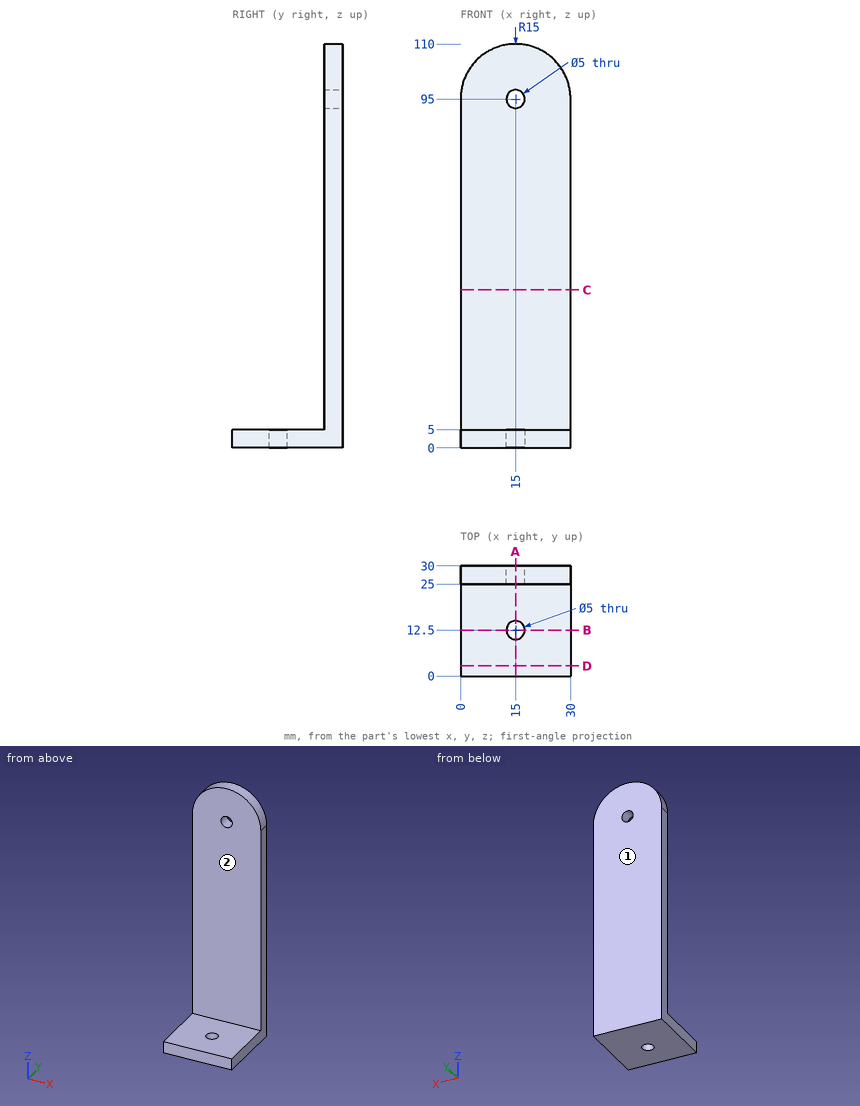
Can you work these out from the drawing? Everything is in mm from the part's minimum corner. A direction names the side the tool comes from. Give positions to 0.01 mm unless a question says otherwise; leave off trailing zeros. Loops run counter-clockwise (first coordinate to the right, second up) from the corner with the lowest first, then second, coordinate; pieces in that order, holes last. Notation, with made-up numbers: M 36,71.25 L 92,71.25 A32 cw 92,100.25 Z; hole C 44.25,77.25 d5. An arc over 180 degrees is marked long. Use CSV: the item, a comma, the result in double quotes. Start each with the question number.
1. On a 3-axis mill with a long thin cutter (end or side, diameter ignored), from which of +Z, -Z, +X, -X, +Y, -Y can I reach the whole of each face in a straight line? I mean the marked faces 1 and 2. Say none if no direction works.
2. For P1, Ø4, axis at x = 14.5, y = 19, coming from the +Z side; P2, Ø6.5, axis at x = 15, z = 95, coming from the -Y side; P3, Ø6, axis at x = 26.5, y = 3, coming from the -Z side, each with a flat end and sliding along its axis, tell me the tip position at first contact or that it passes through.
3. Imagine slicing it at C-C, the plane z = 43. Write out the boundary of the cut face in (x, y).
4. Imagine slicing it at B-B, the plane y = 12.5. Write out the boundary of the cut face in (x, z).
5. Imagine slicing it at D-D, the plane y = 2.75. Write out the boundary of the cut face in (x, z), plus the area to 3 significant figures.
6. Imagine slicing it at A-A, the plane x = 15. Write out the boundary of the cut face in (y, z).
7. If I drill on L1, parallel to Z at x = 15, y = 27.75; L2, parallel to Y at x = 15, z = 2.5; L3, parallel to X at y = 26.7, z = 95, over which ranges is the centre line in solid material (lowest first)?
Response values:
1,face 1,"+Z, -Z, +X, -X, +Y"
1,face 2,"+Z, +X, -X, -Y"
2,P1,"z = 5"
2,P2,"y = 25"
2,P3,"z = 0"
3,outline,"M 0,25 L 30,25 L 30,30 L 0,30 Z"
4,outline,"M 0,0 L 12.5,0 L 12.5,5 L 0,5 Z; M 17.5,0 L 30,0 L 30,5 L 17.5,5 Z"
5,outline,"M 0,0 L 30,0 L 30,5 L 0,5 Z"
5,area,"150 mm^2"
6,outline,"M 0,0 L 10,0 L 10,5 L 0,5 Z; M 15,0 L 30,0 L 30,92.5 L 25,92.5 L 25,5 L 15,5 Z; M 25,97.5 L 30,97.5 L 30,110 L 25,110 Z"
7,L1,"0 to 92.5, 97.5 to 110"
7,L2,"0 to 10, 15 to 30"
7,L3,"0 to 12.5, 17.5 to 30"
